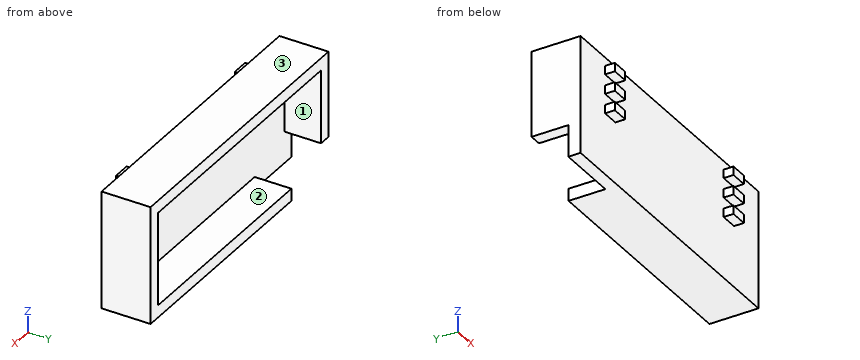
```python
from build123d import *

# Parameters (mm, degrees)
SKETCH1_W           = 120
SKETCH1_H           = 48
BOSS_EXTRUDE1_DEPTH = 5
BOSS_EXTRUDE2_DEPTH = 15
SKETCH3_W           = 7
SKETCH3_H           = 3.5
BOSS_EXTRUDE3_DEPTH = 4


with BuildPart() as part:
    # Sketch1 → Boss-Extrude1 (new body)
    with BuildSketch(Plane(origin=(0, 0, 0), x_dir=(1, 0, 0), z_dir=(0, 1, 0))):
        with Locations((60, 24)):
            Rectangle(SKETCH1_W, SKETCH1_H)
    extrude(amount=BOSS_EXTRUDE1_DEPTH)

    # Sketch2 → Boss-Extrude2 (add)
    with BuildSketch(Plane(origin=(0, 5, 0), x_dir=(1, 0, 0), z_dir=(0, 1, 0))):
        Polygon((120, 48), (25, 48), (25, 43), (115, 43), (115, 5), (5, 5), (5, 35), (0, 35), (0, 0), (120, 0), align=None)
    extrude(amount=BOSS_EXTRUDE2_DEPTH)

    # Sketch3 → Boss-Extrude3 (add)
    with BuildSketch(Plane(origin=(0, 0, 0), x_dir=(-1, 0, 0), z_dir=(0, -1, 0))):
        with Locations((-100, 21.25)):
            Rectangle(SKETCH3_W, SKETCH3_H)
        with Locations((-100, 13.25)):
            Rectangle(SKETCH3_W, SKETCH3_H)
        with Locations((-100, 5.25)):
            Rectangle(SKETCH3_W, SKETCH3_H)
        with Locations((-20, 21.25)):
            Rectangle(SKETCH3_W, SKETCH3_H)
        with Locations((-20, 13.25)):
            Rectangle(SKETCH3_W, SKETCH3_H)
        with Locations((-20, 5.25)):
            Rectangle(SKETCH3_W, SKETCH3_H)
    extrude(amount=BOSS_EXTRUDE3_DEPTH)


solid = part.part
```
Input: part model. Units: mm. Frame: model coordinates. Face numbers are marked on the shaded views. A direction names the side the tool comes from. Coordinates: 2 decimals unless noted, no trailing zeros. Loops run counter-clockwise (first coordinate to the right, second up) from the corner with the lowest first, then second, coordinate; pieces in that order, holes last. Notation, with made-up numbers: (16.25, 52) -> (31.25, 52) arc R36 ccw to (31.25, 89) -> close; hole circle Ø5 at (-28.75, 4.5). An arc over 180 degrees is marked (long way). Use a Markdown table: item, result.
1) Cut plane C-C (x = 67.5). Return the cut outline in (y, z).
Results found:
| item | result |
|---|---|
| outline | (0, -48) -> (20, -48) -> (20, -43) -> (5, -43) -> (5, -5) -> (20, -5) -> (20, 0) -> (0, 0) -> close |
2) Cut plane A-A (y = -1.25). Return the cut outline in (x, z).
Results found:
| item | result |
|---|---|
| outline | (16.5, -23) -> (23.5, -23) -> (23.5, -19.5) -> (16.5, -19.5) -> close; (16.5, -15) -> (23.5, -15) -> (23.5, -11.5) -> (16.5, -11.5) -> close; (16.5, -7) -> (23.5, -7) -> (23.5, -3.5) -> (16.5, -3.5) -> close; (96.5, -23) -> (103.5, -23) -> (103.5, -19.5) -> (96.5, -19.5) -> close; (96.5, -15) -> (103.5, -15) -> (103.5, -11.5) -> (96.5, -11.5) -> close; (96.5, -7) -> (103.5, -7) -> (103.5, -3.5) -> (96.5, -3.5) -> close |
3) Material intervals for line 1 along Z through (x, y) = (78.5, 7.5); line 2 along X through (y, z) = (16, -10.5); line 3 along Y through (x, z) = (34.5, -29.5), sorted ascending. Write a range as from..to.
Results found:
| item | result |
|---|---|
| line 1 | z = -48..-43, -5..0 |
| line 2 | x = 0..5, 115..120 |
| line 3 | y = 0..5 |
4) Cut plane B-B (z = -13). Return the cut outline in (x, y), then the cut area to 3 significant figures.
Results found:
| item | result |
|---|---|
| outline | (0, 0) -> (16.5, 0) -> (16.5, -4) -> (23.5, -4) -> (23.5, 0) -> (96.5, 0) -> (96.5, -4) -> (103.5, -4) -> (103.5, 0) -> (120, 0) -> (120, 20) -> (115, 20) -> (115, 5) -> (5, 5) -> (5, 20) -> (0, 20) -> close |
| area | 806 mm2 |
5) Access query for the marked faces 1, 2 and 3. Directions: +Z, -Z, +X, -X, +Y, -Y. A direction counts if a zero-diameter tool reaches every point of the face in a straight line with its end or side. Return the directions, or none.
Results found:
| item | result |
|---|---|
| face 1 | -Z, +Y |
| face 2 | -X, +Y |
| face 3 | +Z, +X, -X, +Y, -Y |
6) Cut plane D-D (y = 8). Return the cut outline in (x, z).
Results found:
| item | result |
|---|---|
| outline | (0, -35) -> (5, -35) -> (5, -5) -> (115, -5) -> (115, -43) -> (25, -43) -> (25, -48) -> (120, -48) -> (120, 0) -> (0, 0) -> close |
7) Contact query for flat-ended pins moving along their axis: pin 1 (1.8 mm diameter, centred on y = -3, z = -5, fed in from +X); pin 2 (2 mm diameter, centred on x = 100.5, y = -1.5, fed in from +Z); pin 3 (1.8 mm diameter, centred on y = -2.5, z = -21.5, fed in from -X). Output: stop coordinate, or through.
Results found:
| item | result |
|---|---|
| pin 1 | stops at x = 103.5 |
| pin 2 | stops at z = -3.5 |
| pin 3 | stops at x = 16.5 |
